Work out the finished part from the listing and answer in its coordinate system (mm). Face numbers are marked on the shaded views. A direction names the side the tool comes from. Give positions to 0.01 mm unless a question says otherwise; leave off trailing zeros. Loops run counter-clockwise (first coordinate to the right, second up) from the corner with the lowest first, then second, coordinate; pieces in that order, holes last. Notation, with made-up numbers: (1, 55) - (21, 55) arc R22 cw to (21, 82) - close; hole circle Ø9 at (82.5, 4.25). An arc over 180 degrees is marked (long way). Use CSV: the item, a comma, the result in double quotes.
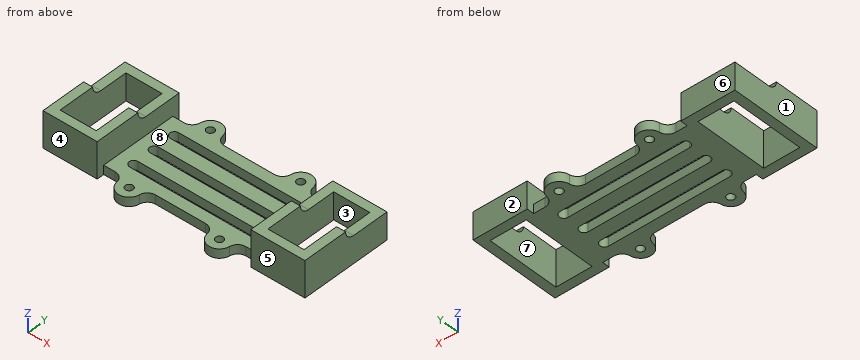
from build123d import *

# Parameters (mm, degrees)
SKETCH2_R           = 0.85
SKETCH2_W           = 8
SKETCH2_H           = 16.2
BOSS_EXTRUDE1_DEPTH = 2
SKETCH6_W           = 12
SKETCH6_H           = 20.2
SKETCH6_W_2         = 8
SKETCH6_H_2         = 16.2
BOSS_EXTRUDE5_DEPTH = 4
BOSS_EXTRUDE6_DEPTH = 2
FILLET1_R           = 2


with BuildPart() as part:
    # Sketch2 → Boss-Extrude1 (new body)
    with BuildSketch(Plane.XY):
        with BuildLine():
            Line((5.527864045, 8.5), (-5.527864045, 8.5))
            ThreePointArc((-5.527864045, 8.5), (-6.861197378, 9.009288015), (-7.515480025, 10.277777778))
            ThreePointArc((-7.515480025, 10.277777778), (-10, 12.5), (-12.484519975, 10.277777778))
            ThreePointArc((-12.484519975, 10.277777778), (-13.138802622, 9.009288015), (-14.472135955, 8.5))
            Line((-14.472135955, 8.5), (-17, 8.5))
            Line((-17, 8.5), (-17, 10.1))
            Line((-17, 10.1), (-29, 10.1))
            Line((-29, 10.1), (-29, 0))
            Line((-29, 0), (-29, -10.1))
            Line((-29, -10.1), (-17, -10.1))
            Line((-17, -10.1), (-17, -8.5))
            Line((-17, -8.5), (-14.472135955, -8.5))
            ThreePointArc((-14.472135955, -8.5), (-13.138802622, -9.009288015), (-12.484519975, -10.277777778))
            ThreePointArc((-12.484519975, -10.277777778), (-10, -12.5), (-7.515480025, -10.277777778))
            ThreePointArc((-7.515480025, -10.277777778), (-6.861197378, -9.009288015), (-5.527864045, -8.5))
            Line((-5.527864045, -8.5), (5.527864045, -8.5))
            ThreePointArc((5.527864045, -8.5), (6.861197378, -9.009288015), (7.515480025, -10.277777778))
            ThreePointArc((7.515480025, -10.277777778), (10, -12.5), (12.484519975, -10.277777778))
            ThreePointArc((12.484519975, -10.277777778), (13.138802622, -9.009288015), (14.472135955, -8.5))
            Line((14.472135955, -8.5), (17, -8.5))
            Line((17, -8.5), (17, -10.1))
            Line((17, -10.1), (29, -10.1))
            Line((29, -10.1), (29, 0))
            Line((29, 0), (29, 10.1))
            Line((29, 10.1), (17, 10.1))
            Line((17, 10.1), (17, 8.5))
            Line((17, 8.5), (14.472135955, 8.5))
            ThreePointArc((14.472135955, 8.5), (13.138802622, 9.009288015), (12.484519975, 10.277777778))
            ThreePointArc((12.484519975, 10.277777778), (10, 12.5), (7.515480025, 10.277777778))
            ThreePointArc((7.515480025, 10.277777778), (6.861197378, 9.009288015), (5.527864045, 8.5))
        make_face()
        with Locations((10, 10)):
            Circle(SKETCH2_R, mode=Mode.SUBTRACT)
        with Locations(Location((-10, 10, 0), (0, 0, 180))):
            Circle(SKETCH2_R, mode=Mode.SUBTRACT)
        with Locations((-10, -10)):
            Circle(SKETCH2_R, mode=Mode.SUBTRACT)
        with Locations(Location((10, -10, 0), (0, 0, 180))):
            Circle(SKETCH2_R, mode=Mode.SUBTRACT)
        with Locations((23, 0)):
            Rectangle(SKETCH2_W, SKETCH2_H, mode=Mode.SUBTRACT)
        with Locations((-23, 0)):
            Rectangle(SKETCH2_W, SKETCH2_H, mode=Mode.SUBTRACT)
        with BuildLine():
            Line((-13.472135955, 6), (13.472135955, 6))
            ThreePointArc((13.472135955, 6), (14.472135955, 5), (13.472135955, 4))
            Line((13.472135955, 4), (-13.472135955, 4))
            ThreePointArc((-13.472135955, 4), (-14.472135955, 5), (-13.472135955, 6))
        make_face(mode=Mode.SUBTRACT)
        with BuildLine():
            Line((13.472135955, -1), (-13.472135955, -1))
            ThreePointArc((-13.472135955, -1), (-14.472135955, 0), (-13.472135955, 1))
            Line((-13.472135955, 1), (13.472135955, 1))
            ThreePointArc((13.472135955, 1), (14.472135955, 0), (13.472135955, -1))
        make_face(mode=Mode.SUBTRACT)
        with BuildLine():
            Line((13.472135955, -6), (-13.472135955, -6))
            ThreePointArc((-13.472135955, -6), (-14.472135955, -5), (-13.472135955, -4))
            Line((-13.472135955, -4), (13.472135955, -4))
            ThreePointArc((13.472135955, -4), (14.472135955, -5), (13.472135955, -6))
        make_face(mode=Mode.SUBTRACT)
    extrude(amount=BOSS_EXTRUDE1_DEPTH)

    # Sketch6 → Boss-Extrude5 (add)
    # profile 1 of 2: a face of its own
    with BuildSketch(Plane.XY.offset(2)):
        with Locations((-23, 0)):
            Rectangle(SKETCH6_W, SKETCH6_H)
        with Locations((-23, 0)):
            Rectangle(SKETCH6_W_2, SKETCH6_H_2, mode=Mode.SUBTRACT)
    # profile 2 of 2: a face of its own
    with BuildSketch(Plane.XY.offset(2)):
        with Locations((23, 0)):
            Rectangle(SKETCH6_W, SKETCH6_H)
        with Locations((23, 0)):
            Rectangle(SKETCH6_W_2, SKETCH6_H_2, mode=Mode.SUBTRACT)
    extrude(amount=BOSS_EXTRUDE5_DEPTH)

    # Sketch7 → Boss-Extrude6 (add)
    with BuildSketch(Plane.XY.offset(6)):
        Polygon((17, -0.1), (19, -0.1), (19, -8.1), (27, -8.1), (27, -0.1), (29, -0.1), (29, -10.1), (17, -10.1), align=None)
        Polygon((-17, -10.1), (-17, -0.1), (-19, -0.1), (-19, -8.1), (-27, -8.1), (-27, -0.1), (-29, -0.1), (-29, -10.1), align=None)
    extrude(amount=BOSS_EXTRUDE6_DEPTH)

    # Fillet1
    fillet1_edges = [part.edges().sort_by_distance(p)[0] for p in [
        (28, -0.1, 6),
        (18, -0.1, 6),
        (-18, -0.1, 6),
        (-28, -0.1, 6),
    ]]
    fillet(fillet1_edges, radius=FILLET1_R - 0.0001)  # a hair under: the kernel refuses the full size


solid = part.part
Item 1: Given P1, Ø1, axis at x = -15.5, z = 1, coming from the +Y side; P2, Ø12, axis at x = -11.5, y = -3.5, coming from the +Z side; P3, Ø2, axis at x = 2.5, z = 0.5, coming from the -Y side; P4, Ø2, axis at x = 10, y = -10, coming from the +Z side, each flat-ended and moving along its own axis, determine where each tip first touches the part or whether it passes through.
Determined:
P1,"stops at y = 8.5"
P2,"stops at z = 8"
P3,"stops at y = -8.5"
P4,"stops at z = 2"
Item 2: Find the intervals of material crossed by line 1 (X direction, y = 4, z = 2.25); line 2 (Y direction, x = -22, z = 5); line 3 (X direction, y = -8.5, z = 3.5), in increasing order.
Determined:
line 1,"x = -29 to -27, -19 to -17, 17 to 19, 27 to 29"
line 2,"y = -10.1 to -8.1, 8.1 to 10.1"
line 3,"x = -29 to -17, 17 to 29"
Item 3: A cutting plane is placed at A-A on x = -4. Determine the outline of the cut face in (y, z), and give its area (3 significant figures).
Determined:
outline,"(-8.5, 0) - (-6, 0) - (-6, 2) - (-8.5, 2) - close; (-4, 0) - (-1, 0) - (-1, 2) - (-4, 2) - close; (1, 0) - (4, 0) - (4, 2) - (1, 2) - close; (6, 0) - (8.5, 0) - (8.5, 2) - (6, 2) - close"
area,"22.0 mm²"
Item 4: The mould has two halves that part along X. Classify the marked faces 1, 2 and 3: pulls with the +X half, pulls with the -X half, needs draft (parallel to the pull), parting line crosses it, or undercut.
Determined:
face 1,"pulls with the -X half"
face 2,"needs draft"
face 3,"undercut"
Item 5: For the marked faces 4, 5, 6, 7 and 8, determine the directions among +Z, -Z, +X, -X, +Y, -Y from which every point of the face is accessible in a straight line to the end or side of a thin tool.
Determined:
face 4,"+Z, -Z, -X, -Y"
face 5,"+Z, -Z, +X, -Y"
face 6,"+Z, -Z, -X, +Y"
face 7,"+Z, -Z"
face 8,"+Z, +Y, -Y"
Item 6: A cutting plane is placed at D-D on y = -7.25. Determine the outline of the cut face in (x, z), and give its area (3 significant figures).
Determined:
outline,"(-29, 0) - (-27, 0) - (-27, 8) - (-29, 8) - close; (-19, 0) - (19, 0) - (19, 8) - (17, 8) - (17, 2) - (-17, 2) - (-17, 8) - (-19, 8) - close; (27, 0) - (29, 0) - (29, 8) - (27, 8) - close"
area,"132 mm²"
Item 7: A cutting plane is placed at C-C on x = 10. Determine the outline of the cut face in (y, z).
Determined:
outline,"(-12.5, 0) - (-10.85, 0) - (-10.85, 2) - (-12.5, 2) - close; (-9.15, 0) - (-6, 0) - (-6, 2) - (-9.15, 2) - close; (-4, 0) - (-1, 0) - (-1, 2) - (-4, 2) - close; (1, 0) - (4, 0) - (4, 2) - (1, 2) - close; (6, 0) - (9.15, 0) - (9.15, 2) - (6, 2) - close; (10.85, 0) - (12.5, 0) - (12.5, 2) - (10.85, 2) - close"
Item 8: A cutting plane is placed at B-B on y = 5. Determine the outline of the cut face in (x, z), and give its area (3 significant figures).
Determined:
outline,"(-29, 0) - (-27, 0) - (-27, 6) - (-29, 6) - close; (-19, 0) - (-14.47, 0) - (-14.47, 2) - (-17, 2) - (-17, 6) - (-19, 6) - close; (14.47, 0) - (19, 0) - (19, 6) - (17, 6) - (17, 2) - (14.47, 2) - close; (27, 0) - (29, 0) - (29, 6) - (27, 6) - close"
area,"58.1 mm²"
